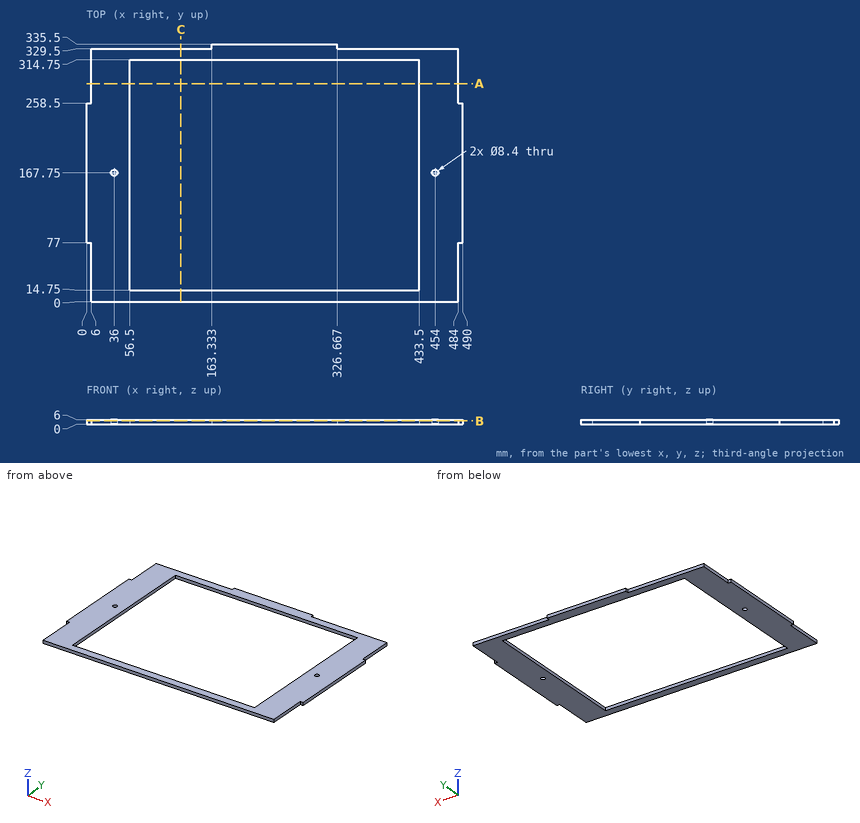
Part print with two shaded views. Sizes in mm from the minimum x, y, z corner. Coordinates: 2 decimals unless noted, no trailing zeros. Write each loop counter-clockwise with the first axis right and the second up, starting at its lowest first coordinate (ties: lowest second). Pieces come first, ordered by that corner, then holes. Notation, with made-up numbers: (62, 4) - (91, 4) arc R14 cw to (91, 18) - close; hole circle Ø4 at (33.5, -12). An arc over 180 degrees is marked (long way). One line per item, written item: value. Start each with the question number.
1. Slice it at B-B (z = 4.3). Write the cut outline in (x, y), plus the area to 4 significant figures.
2. Flat gauge pins, fed straight in: pin 1 (1.8 mm diameter, centred on x = 99, z = 2, fed in from +Y); pin 2 (3 mm diameter, centred on x = 3.5, z = 4, fed in from +Y); pin 3 (3 mm diameter, centred on x = 2.5, z = 4, fed in from -Y); pin 4 (7.5 mm diameter, centred on x = 36, y = 167.75, fed in from +Z). Where does each tip first touch, or does it go through?
3. Slice it at C-C (x = 123). Write the cut outline in (y, z).
4. Slice it at A-A (y = 284). Write the cut outline in (x, z).
5. Probe line 1 (Y direction, x = 220, z = 5.8); line 2 (X direction, y = 100, z = 1.6); line 3 (X direction, y = 64, z = 4.45). List the from-to ranges inside material, lowest first. Write a range as from..to.
Answers below:
1. outline: (0, 77) - (6, 77) - (6, 0) - (484, 0) - (484, 77) - (490, 77) - (490, 258.5) - (484, 258.5) - (484, 329.5) - (326.67, 329.5) - (326.67, 335.5) - (163.33, 335.5) - (163.33, 329.5) - (6, 329.5) - (6, 258.5) - (0, 258.5) - close; hole circle Ø8.4 at (36, 167.75); hole (56.5, 14.75) - (433.5, 14.75) - (433.5, 314.75) - (56.5, 314.75) - close; hole circle Ø8.4 at (454, 167.75)
1. area: 47,450 mm^2
2. pin 1: stops at y = 329.5
2. pin 2: stops at y = 258.5
2. pin 3: stops at y = 77
2. pin 4: passes through
3. outline: (0, 0) - (14.75, 0) - (14.75, 6) - (0, 6) - close; (314.75, 0) - (329.5, 0) - (329.5, 6) - (314.75, 6) - close
4. outline: (6, 0) - (56.5, 0) - (56.5, 6) - (6, 6) - close; (433.5, 0) - (484, 0) - (484, 6) - (433.5, 6) - close
5. line 1: y = 0..14.75, 314.75..335.5
5. line 2: x = 0..56.5, 433.5..490
5. line 3: x = 6..56.5, 433.5..484
